Input: part model. Units: mm. Frame: model coordinates. Face numbers are marked on the shaded views. A direction names the side the tool comes from. Round coordinates to 2 decimals unless told otherwise and drop trailing zeros. Order: outer loops, then holes, each group sorted by start corner. A loop starts at its lowest first (then second) coordinate and runs counter-clockwise, first axis right, second up. Notation, with made-up numbers: (87.25, 72.5) -> (119.25, 72.5) arc R17 ccw to (119.25, 93.5) -> close; hole circle Ø5 at (-1, 12). An arc over 180 degrees is marked (long way). Answer as CSV lines item,"result". Start each with the question number.
1) Section query B-B, the plane z = 28.5. Output: boundary loops of the cut face in (x, y).
2) Section query C-C, the plane x = 26.5. Output: boundary loops of the cut face in (y, z), and give its area (3 significant figures).
3) Mould query, pull axis X, two halves, no side actions, for the marked faces 5, 6, 7 and 8. Classes: +X half, -X half, draft (parallel to the pull), parting line (faces both ways), or undercut.
4) Access query for the marked faces 1, 2, 3 and 4. Directions: +Z, -Z, +X, -X, +Y, -Y. A direction counts if a zero-diameter tool reaches every point of the face in a straight line with its end or side. Return the directions, or none.
5) Section query D-D, the plane z = 19. Output: boundary loops of the cut face in (x, y), and give its area (3 significant figures).
6) First-contact query: P1, Ø4, axis at x = -27.5, y = -2, coming from the +Z side; P2, Ø1, axis at y = 4.5, z = 21, coming from the -X side; P3, Ø5, axis at y = -0.5, z = 15.5, coming from the -X side. Flat tips, straight axial feed; report the tip coordinate or a pass-through.
7) Section query A-A, the plane y = 1.5. Output: boundary loops of the cut face in (x, z).
8) Line query: L1, parallel to Z at x = -21, y = 4.25; L2, parallel to X at y = 0.25, z = 29; L3, parallel to X at y = 5, z = -27. Output: solid intervals per line, ascending.
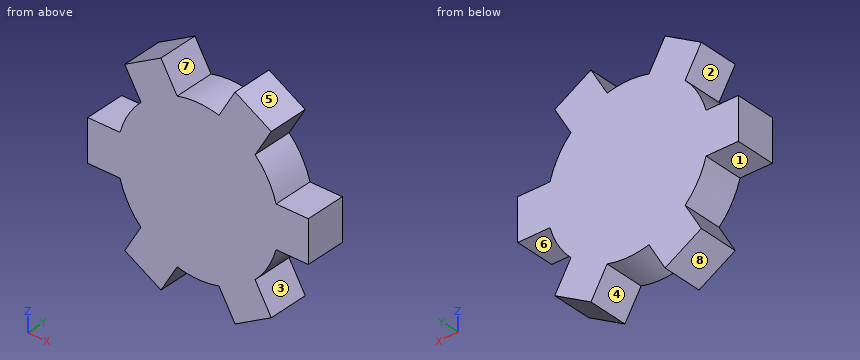
```python
from build123d import *

# Parameters (mm, degrees)
F0_R     = 25.4
F1_DEPTH = 6.35
F3_DEPTH = 12.7
F5_COUNT = 6


with BuildPart() as f1:
    # F0 (on Front) → F1 (new body, symmetric)
    with BuildSketch(Plane.XZ):
        Circle(F0_R)
    extrude(amount=F1_DEPTH, both=True)

    # F2 (on face) → F3 (join)
    with BuildSketch(Plane.XZ.offset(6.35)):
        Polygon((24.534516, 6.574004), (0, 0), (24.534516, 0), align=None)
        Polygon((24.534516, 0), (0, 0), (24.534516, -6.574004), align=None)
        with BuildLine():
            Line((25.4, 0), (24.534516, 0))
            Line((24.534516, 0), (24.534516, -6.574004))
            ThreePointArc((24.534516, -6.574004), (25.182699, -3.315365), (25.4, 0))
        make_face()
        with BuildLine():
            Line((24.534516, 6.574004), (24.534516, 0))
            Line((24.534516, 0), (25.4, 0))
            ThreePointArc((25.4, 0), (25.182699, 3.315365), (24.534516, 6.574004))
        make_face()
        with BuildLine():
            Line((34.694516, 6.574004), (24.534516, 6.574004))
            ThreePointArc((24.534516, 6.574004), (25.182699, 3.315365), (25.4, 0))
            ThreePointArc((25.4, 0), (25.182699, -3.315365), (24.534516, -6.574004))
            Line((24.534516, -6.574004), (34.694516, -6.574004))
            Line((34.694516, -6.574004), (34.694516, 6.574004))
        make_face()
    extrude(amount=-F3_DEPTH)

    # F5: F1 ×6 about axis
    f5_axis = Axis((0, -14.801851, 0), (0, 1, 0))


with BuildPart() as f1_1:
    add(f1.part)
    for i in range(1, F5_COUNT):
        add(f1.part.rotate(f5_axis, i * 360 / F5_COUNT))


solid = f1_1.part
```
Findings:
1,outline,"(-20.03, -6.35) -> (-8.86, -6.35) -> (-8.86, 6.35) -> (-20.03, 6.35) -> close; (8.86, -6.35) -> (20.03, -6.35) -> (20.03, 6.35) -> (8.86, 6.35) -> close"
2,outline,"(-6.35, -6.57) -> (6.35, -6.57) -> (6.35, 6.57) -> (-6.35, 6.57) -> close"
2,area,"167 mm^2"
3,face 5,"+X half"
3,face 6,"draft"
3,face 7,"undercut"
3,face 8,"-X half"
4,face 1,"-Z, -X, +Y, -Y"
4,face 2,"-X, +Y, -Y"
4,face 3,"+X, +Y, -Y"
4,face 4,"-Z, +Y, -Y"
5,outline,"(-18.56, -6.35) -> (18.56, -6.35) -> (18.56, 6.35) -> (-18.56, 6.35) -> close"
5,area,"471 mm^2"
6,P1,"stops at z = 6.57"
6,P2,"stops at x = -20"
6,P3,"stops at x = -21.82"
7,outline,"(-34.69, -6.57) -> (-24.53, -6.57) arc R25.4 ccw to (-17.96, -17.96) -> (-23.04, -26.76) -> (-11.65, -33.33) -> (-6.57, -24.53) arc R25.4 ccw to (6.57, -24.53) -> (11.65, -33.33) -> (23.04, -26.76) -> (17.96, -17.96) arc R25.4 ccw to (24.53, -6.57) -> (34.69, -6.57) -> (34.69, 6.57) -> (24.53, 6.57) arc R25.4 ccw to (17.96, 17.96) -> (23.04, 26.76) -> (11.65, 33.33) -> (6.57, 24.53) arc R25.4 ccw to (-6.57, 24.53) -> (-11.65, 33.33) -> (-23.04, 26.76) -> (-17.96, 17.96) arc R25.4 ccw to (-24.53, 6.57) -> (-34.69, 6.57) -> close"
8,L1,"z = -27.94 to -23.23, -14.29 to 14.29, 23.23 to 27.94"
8,L2,"x = -19.16 to -9.15, 9.15 to 19.16"
8,L3,"x = -22.62 to -8, 8 to 22.62"
